Build history of the part. All positions in model axes, mm. Round coordinates to 2 decimals unless told otherwise and drop trailing zeros. Loops run counter-clockwise (first coordinate to the right, second up) from the corner with the lowest first, then second, coordinate; pieces in that order, holes last.
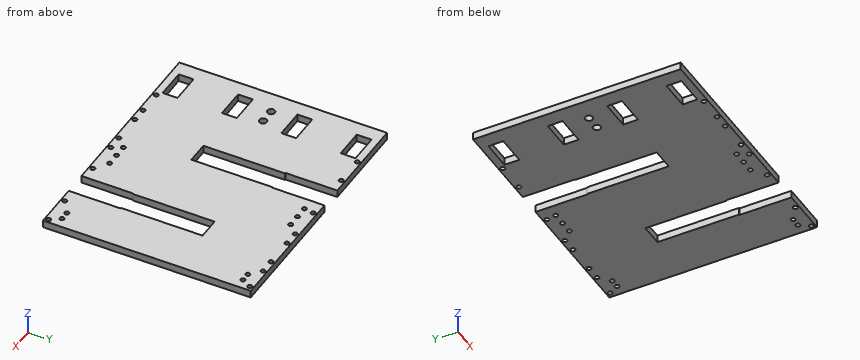
from build123d import *

# Parameters (mm, degrees)
SKETCH_1_W          = 140
SKETCH_1_H          = 140
EXTRUDE_1_DEPTH     = 5
SKETCH_3_W          = 30
SKETCH_3_H          = 140
EXTRUDE_2_DEPTH     = 5
CUT_EXTRUDE_9_DEPTH = 10
SKETCH_4_W          = 20
SKETCH_4_H          = 10
CUT_EXTRUDE_2_DEPTH = 10
SKETCH_6_R          = 1.5
CUT_EXTRUDE_6_DEPTH = 31
CUT_EXTRUDE_7_DEPTH = 10
SKETCH_8_R          = 1.5
CUT_EXTRUDE_8_DEPTH = 10


with BuildPart() as part:
    # 스케치1 → 보스-돌출1 (new body)
    with BuildSketch(Plane.XY):
        Rectangle(SKETCH_1_W, SKETCH_1_H)
    extrude(amount=EXTRUDE_1_DEPTH)

    # 스케치3 → 보스-돌출2 (add)
    with BuildSketch(Plane.XY.offset(5)):
        with Locations((-85, 0)):
            Rectangle(SKETCH_3_W, SKETCH_3_H)
    extrude(amount=-EXTRUDE_2_DEPTH)

    # 스케치2 → 컷-돌출9 (cut)
    with BuildSketch(Plane.XY.offset(5)):
        Polygon((-38, 70), (-22, 70), (-22, 35), (-22.5, 35), (-22.5, -20), (-37.5, -20), (-37.5, 35), (-38, 35), align=None)
        Polygon((22, -70), (22, -35), (22.5, -35), (22.5, 20), (37.5, 20), (37.5, -35), (38, -35), (38, -70), align=None)
    extrude(amount=-CUT_EXTRUDE_9_DEPTH, mode=Mode.SUBTRACT)

    # 스케치4 → 컷-돌출2 (cut)
    with BuildSketch(Plane(origin=(0, 0, 0), x_dir=(-1, 0, 0), z_dir=(0, 0, -1))):
        with Locations((80, 60)):
            Rectangle(SKETCH_4_W, SKETCH_4_H)
        with Locations((80, 20)):
            Rectangle(SKETCH_4_W, SKETCH_4_H)
        with Locations((80, -20)):
            Rectangle(SKETCH_4_W, SKETCH_4_H)
        with Locations((80, -60)):
            Rectangle(SKETCH_4_W, SKETCH_4_H)
    extrude(amount=-CUT_EXTRUDE_2_DEPTH, mode=Mode.SUBTRACT)

    # 스케치6 → 컷-돌출6 (cut)
    with BuildSketch(Plane.XY.offset(5)):
        with Locations((-10, -67.5)):
            Circle(SKETCH_6_R)
        with Locations((-20, -67.5)):
            Circle(SKETCH_6_R)
        with Locations((-66.5, -67.5)):
            Circle(SKETCH_6_R)
        with Locations((-67.5, 67.5)):
            Circle(SKETCH_6_R)
        with Locations((-47.5, 67.5)):
            Circle(SKETCH_6_R)
        with Locations((-12.5, 67.5)):
            Circle(SKETCH_6_R)
        with Locations((10, 67.5)):
            Circle(SKETCH_6_R)
        with Locations((20, 67.5)):
            Circle(SKETCH_6_R)
        with Locations((40, 67.5)):
            Circle(SKETCH_6_R)
        with Locations((66.5, 67.5)):
            Circle(SKETCH_6_R)
        with Locations((67.5, -67.5)):
            Circle(SKETCH_6_R)
        with Locations((47.5, -67.5)):
            Circle(SKETCH_6_R)
        with Locations((12.5, -67.5)):
            Circle(SKETCH_6_R)
        with Locations((-40, -67.5)):
            Circle(SKETCH_6_R)
        with Locations((-50, -67.5)):
            Circle(SKETCH_6_R)
        with Locations((50, 67.5)):
            Circle(SKETCH_6_R)
    extrude(amount=-CUT_EXTRUDE_6_DEPTH, mode=Mode.SUBTRACT)

    # 스케치7 → 컷-돌출7 (cut)
    with BuildSketch(Plane.XY.offset(5)):
        with BuildLine():
            ThreePointArc((-82.5, 0), (-85, 2.5), (-87.5, 0))
            Line((-87.5, 0), (-82.5, 0))
        make_face()
        with BuildLine():
            Line((-82.5, 0), (-87.5, 0))
            ThreePointArc((-87.5, 0), (-85, -2.5), (-82.5, 0))
        make_face()
        with BuildLine():
            ThreePointArc((-72.5, 0), (-75, 2.5), (-77.5, 0))
            Line((-77.5, 0), (-72.5, 0))
        make_face()
        with BuildLine():
            Line((-72.5, 0), (-77.5, 0))
            ThreePointArc((-77.5, 0), (-75, -2.5), (-72.5, 0))
        make_face()
    extrude(amount=-CUT_EXTRUDE_7_DEPTH, mode=Mode.SUBTRACT)

    # 스케치8 → 컷-돌출8 (cut)
    with BuildSketch(Plane(origin=(0, 0, 0), x_dir=(-1, 0, 0), z_dir=(0, 0, -1))):
        with BuildLine():
            ThreePointArc((-58.5, 61), (-57, 59.5), (-55.5, 61))
            Line((-55.5, 61), (-58.5, 61))
        make_face()
        with BuildLine():
            Line((-58.5, 61), (-55.5, 61))
            ThreePointArc((-55.5, 61), (-57, 62.5), (-58.5, 61))
        make_face()
        with BuildLine():
            ThreePointArc((-5, 61), (-3.5, 59.5), (-2, 61))
            Line((-2, 61), (-5, 61))
        make_face()
        with BuildLine():
            Line((-5, 61), (-2, 61))
            ThreePointArc((-2, 61), (-3.5, 62.5), (-5, 61))
        make_face()
        with BuildLine():
            ThreePointArc((-64.5, 61), (-63, 59.5), (-61.5, 61))
            Line((-61.5, 61), (-64.5, 61))
        make_face()
        with BuildLine():
            Line((-64.5, 61), (-61.5, 61))
            ThreePointArc((-61.5, 61), (-63, 62.5), (-64.5, 61))
        make_face()
        with Locations((13.5, -61)):
            Circle(SKETCH_8_R)
        with Locations((5, -61)):
            Circle(SKETCH_8_R)
        with BuildLine():
            ThreePointArc((12, 61), (13.5, 59.5), (15, 61))
            Line((15, 61), (12, 61))
        make_face()
        with BuildLine():
            Line((12, 61), (15, 61))
            ThreePointArc((15, 61), (13.5, 62.5), (12, 61))
        make_face()
        with BuildLine():
            ThreePointArc((3.5, 61), (5, 59.5), (6.5, 61))
            Line((6.5, 61), (3.5, 61))
        make_face()
        with BuildLine():
            Line((3.5, 61), (6.5, 61))
            ThreePointArc((6.5, 61), (5, 62.5), (3.5, 61))
        make_face()
        with Locations((-3.5, -61)):
            Circle(SKETCH_8_R)
        with Locations((-63, -61)):
            Circle(SKETCH_8_R)
        with Locations((-57, -61)):
            Circle(SKETCH_8_R)
    extrude(amount=-CUT_EXTRUDE_8_DEPTH, mode=Mode.SUBTRACT)


solid = part.part
(1) Slice it at B-B on x = -85. List the corners of the cut face in (y, z).
Responses:
outline: (-70, 0) - (-65, 0) - (-65, 5) - (-70, 5) - close; (-55, 0) - (-25, 0) - (-25, 5) - (-55, 5) - close; (-15, 0) - (-2.5, 0) - (-2.5, 5) - (-15, 5) - close; (2.5, 0) - (15, 0) - (15, 5) - (2.5, 5) - close; (25, 0) - (55, 0) - (55, 5) - (25, 5) - close; (65, 0) - (70, 0) - (70, 5) - (65, 5) - close
(2) Probe line 1 (X direction, y = 17, z = 2.4); line 2 (X direction, y = 5, z = 2.05); line 3 (Y direction, x = -5, z = 2.4). List the from-to ranges inside material, lowest first.
Responses:
line 1: x = -100 to -90, -70 to -37.5, -22.5 to 22.5, 37.5 to 70
line 2: x = -100 to -37.5, -22.5 to 22.5, 37.5 to 70
line 3: y = -70 to -62.5, -59.5 to 59.5, 62.5 to 70
(3) Slice it at A-A on y = 10. List the corners of the cut face in (x, z), plus the area to 3 significant figures.
Responses:
outline: (-100, 0) - (-37.5, 0) - (-37.5, 5) - (-100, 5) - close; (-22.5, 0) - (22.5, 0) - (22.5, 5) - (-22.5, 5) - close; (37.5, 0) - (70, 0) - (70, 5) - (37.5, 5) - close
area: 700 mm2
(4) Slice it at D-D on z = 1.35. Count the separate pieces of the cut face and the enclosed holes in it, plus the area to 3 significant figures.
Responses:
separate pieces: 1
enclosed holes: 32
area: 20,000 mm2
(5) Slice it at C-C on y = -40. List the corners of the cut face in (x, z).
Responses:
outline: (-100, 0) - (22, 0) - (22, 5) - (-100, 5) - close; (38, 0) - (70, 0) - (70, 5) - (38, 5) - close
